Autodesk Inventor part; units mm, degrees
ref_plane "YZ Plane" through (0, 0, 0) normal (1, 0, 0) x (0, 1, 0)
ref_plane "XZ Plane" through (0, 0, 0) normal (0, 1, 0) x (-1, 0, 0)
ref_plane "XY Plane" through (0, 0, 0) normal (0, 0, 1) x (1, 0, 0)
sketch "Sketch1" plane through (0, 0, 0) normal (0, 0, 1) x (1, 0, 0)
  line L0 (21.5871, 13.6345) -> (17.0871, 18.1345)
  line L1 (17.0871, 18.1345) -> (-16.7129, 18.1345)
  line L2 (-16.7129, 18.1345) -> (-21.2129, 13.6345)
  line L3 (-21.0966, 13.6345) -> (-21.0966, -20.1655)
  line L4 (21.4709, -20.1655) -> (21.4709, 13.6345)
  line L5 (21.4709, -20.1655) -> (17.0871, -24.4078)
  line L6 (-16.7129, -24.4078) -> (17.0871, -24.4078)
  line L7 (-16.7129, -24.4078) -> (-21.0966, -20.1655)
  line L8 (-24.7129, -28.1655) -> (-24.7129, 13.6345) construction
  line L9 (25.0871, -28.1655) -> (-24.7129, -28.1655) construction
  line L10 (25.0871, -28.1655) -> (25.0871, 13.6345) construction
  line L11 (17.0871, 21.6345) -> (-16.7129, 21.6345) construction
  line L12 (-21.0552, -20.0655) -> (-16.6129, -24.5078)
  line L13 (-16.6129, -24.5078) -> (-16.6129, -28.1655)
  line L14 (-16.6129, -28.1655) -> (17.0871, -28.1655)
  line L15 (25.0871, -20.0655) -> (21.4295, -20.0655)
  line L16 (25.0871, 13.5345) -> (25.0871, -20.0655)
  line L17 (21.4295, 13.5345) -> (25.0871, 13.5345)
  line L18 (21.4295, 13.5345) -> (16.9871, 17.9768)
  line L19 (16.9871, 17.9768) -> (16.9871, 21.6345)
  line L20 (16.9871, 21.6345) -> (-16.6129, 21.6345)
  line L21 (-16.6129, 21.6345) -> (-16.6129, 17.9768)
  line L22 (-16.6129, 17.9768) -> (-21.0552, 13.5345)
  line L23 (-24.7129, 13.5345) -> (-21.0552, 13.5345)
  line L24 (-24.7129, -20.0655) -> (-24.7129, 13.5345)
  line L25 (-21.0552, -20.0655) -> (-24.7129, -20.0655)
  line L26 (-12.3129, -23.2655) -> (12.6871, -23.2655)
  line L27 (12.6871, -23.2655) -> (12.6871, 16.7345)
  line L28 (-12.3129, 16.7345) -> (12.6871, 16.7345)
  line L29 (-12.3129, -23.2655) -> (-12.3129, 16.7345)
  line L30 (14.6871, -25.2655) -> (-14.3129, -25.2655) construction
  line L31 (-14.3129, -25.2655) -> (-14.3129, 18.7345) construction
  line L32 (-14.3129, 18.7345) -> (14.6871, 18.7345) construction
  line L33 (14.6871, 18.7345) -> (14.6871, -25.2655) construction
  line L34 (-17.3129, 21.7345) -> (17.6871, 21.7345) construction
  line L35 (17.6871, 21.7345) -> (17.6871, -28.2655) construction
  line L36 (17.6871, -28.2655) -> (-17.3129, -28.2655) construction
  line L37 (-17.3129, -28.2655) -> (-17.3129, 21.7345) construction
  line L38 (-14.3129, -23.2655) -> (-14.3129, -25.2655)
  line L39 (-14.3129, -25.2655) -> (14.6871, -25.2655)
  line L40 (14.6871, -25.2655) -> (14.6871, -20.0655)
  line L41 (14.6871, -20.0655) -> (17.6871, -20.0655)
  line L42 (17.6871, -20.0655) -> (17.6871, 13.5345)
  line L43 (17.6871, 13.5345) -> (14.6871, 13.5345)
  line L44 (14.6871, 13.5345) -> (14.6871, 18.7345)
  line L45 (14.6871, 18.7345) -> (-14.3129, 18.7345)
  line L46 (-14.3129, 18.7345) -> (-14.3129, 13.5345)
  line L47 (-14.3129, 13.5345) -> (-17.3129, 13.5345)
  line L48 (-17.3129, 13.5345) -> (-17.3129, -20.0655)
  line L49 (-17.3129, -20.0655) -> (-14.3129, -20.0655)
  line L50 (-14.3129, -20.0655) -> (-14.3129, -23.2655)
  line L51 (-16.6129, -28.1655) -> (17.0871, -28.1655)
  line L52 (16.9871, -28.1655) -> (16.9871, -24.3509)
  line L53 (16.9871, -24.3509) -> (21.2726, -20.0655)
  line L54 (21.2726, -20.0655) -> (21.4295, -20.0655)
  point P0 (14.2, -44.8454)
  point P1 (16.9871, 19.8057)
  dimension "d74" = 2
  dimension "d75" = 5
  dimension "d76" = 135
extrude "Extrusion1" add sketch "Sketch1" along normal blind 8 contours L19 L18 L17 L4 L15 L54 L53 L52 L6 L40 L41 L42 L43 L44 L1 | L1 L44 L45 L46 L21 L20 L19 | L44 L43 L42 L41 L40 L6 L38 L50 L49 L48 L47 L46 L1 | L1 L46 L45 L44 | L46 L47 L48 L49 L50 L38 L6 L12 L25 L3 L23 L22 L21 L1 | L17 L16 L15 L4 | L3 L25 L24 L23 | L40 L39 L38 L6 | L6 L52 L14 L13 L12 L38 L39 L40 | L29 L28 L27 L26
sketch "Skizze7" plane through (0, 0, 8) normal (0, 0, 1) x (1, 0, 0)
  line L0 (-21.0552, -20.0655) -> (-16.6129, -24.5078)
  line L1 (-16.6129, -24.5078) -> (-16.6129, -28.1655)
  line L2 (-16.6129, -28.1655) -> (16.9871, -28.1655) construction
  line L3 (16.9871, -28.1655) -> (16.9871, -24.3509)
  line L4 (16.9871, -24.3509) -> (21.2726, -20.0655)
  line L5 (21.2726, -20.0655) -> (25.0871, -20.0655)
  line L6 (25.0871, -20.0655) -> (25.0871, 13.5345) construction
  line L7 (25.0871, 13.5345) -> (21.4295, 13.5345)
  line L8 (21.4295, 13.5345) -> (16.9871, 17.9768)
  line L9 (16.9871, 17.9768) -> (16.9871, 21.6345)
  line L10 (16.9871, 21.6345) -> (-16.6129, 21.6345) construction
  line L11 (-16.6129, 21.6345) -> (-16.6129, 17.9768)
  line L12 (-16.6129, 17.9768) -> (-21.0552, 13.5345)
  line L13 (-21.0552, 13.5345) -> (-24.7129, 13.5345)
  line L14 (-24.7129, 13.5345) -> (-24.7129, -20.0655) construction
  line L15 (-24.7129, -20.0655) -> (-21.0552, -20.0655)
  line L16 (-16.8129, 21.8345) -> (17.1871, 21.8345) construction
  line L17 (17.1871, 21.8345) -> (17.1871, 18.0597)
  line L18 (17.1871, 18.0597) -> (21.5123, 13.7345)
  line L19 (21.5123, 13.7345) -> (25.2871, 13.7345)
  line L20 (25.2871, 13.7345) -> (25.2871, -20.2655) construction
  line L21 (25.2871, -20.2655) -> (21.3554, -20.2655)
  line L22 (21.3554, -20.2655) -> (17.1871, -24.4338)
  line L23 (17.1871, -24.4338) -> (17.1871, -28.3655)
  line L24 (17.1871, -28.3655) -> (-16.8129, -28.3655) construction
  line L25 (-16.8129, -28.3655) -> (-16.8129, -24.5907)
  line L26 (-16.8129, -24.5907) -> (-21.1381, -20.2655)
  line L27 (-21.1381, -20.2655) -> (-24.9129, -20.2655)
  line L28 (-24.9129, -20.2655) -> (-24.9129, 13.7345) construction
  line L29 (-24.9129, 13.7345) -> (-21.1381, 13.7345)
  line L30 (-21.1381, 13.7345) -> (-16.8129, 18.0597)
  line L31 (-16.8129, 18.0597) -> (-16.8129, 21.8345)
  line L32 (-21.0552, 13.5345) -> (-24.7129, 13.5345)
  line L33 (-24.7129, 13.5345) -> (-24.7129, 13.7345)
  line L34 (-16.6129, 21.6345) -> (-16.6129, 17.9768)
  line L35 (-16.6129, 21.6345) -> (-16.8129, 21.6345)
  line L36 (25.0871, -20.0655) -> (25.0871, 13.5345)
  line L37 (25.0871, 13.5345) -> (25.0871, 13.7345)
  line L38 (16.9871, 21.6345) -> (17.1871, 21.6345)
  line L39 (16.9871, -28.1655) -> (17.1871, -28.1655)
  line L40 (25.0871, -20.0655) -> (25.0871, -20.2655)
  line L41 (-16.6129, -28.1655) -> (-16.8129, -28.1655)
  line L42 (-24.7129, -20.0655) -> (-24.7129, -20.2655)
  dimension "d94" = 0.2
extrude "IM_offset" add sketch "Skizze7" against normal up to surface (8 mm away)
sketch "Sketch8" plane through (-1.6003, 36.8471, 0) normal (0.7071, 0.7071, 0) x (0.7071, -0.7071, 0)
  arc A0 (21.9778, -0.9777) -> (37.2778, -0.9777) centre (29.6278, -0.9777) ccw
  line L0 (21.9778, -0.9777) -> (37.2778, -0.9777) construction
  line L1 (21.9778, -0.9777) -> (37.2778, -0.9777) construction
  line L2 (21.9778, -0.9777) -> (37.2778, -0.9777)
  point P0 (27.1864, 0)
  point P1 (29.6278, -1.0154)
  dimension "d98" = 15.3
  dimension "d99" = 0
  dimension "d100" = 7.65
extrude "Extrusion7" cut sketch "Sketch8" against normal blind 45 and the other way blind 22.5
sketch "Sketch9" plane through (0, 0, 8) normal (0, 0, 1) x (1, 0, 0)
  line L0 (17.1871, 21.6345) -> (-16.8129, 21.6345)
  line L1 (-24.7129, 13.7345) -> (-24.7129, -20.2655)
  line L2 (17.1871, -28.1655) -> (-16.8129, -28.1655)
  line L3 (25.0871, -20.0655) -> (25.0871, 13.7345)
  circle A0 centre (0.1871, -3.187) radius 27.0445
  circle A1 centre (0.1871, -3.187) radius 15
  line L4 (-16.8129, 21.6345) -> (-16.8129, 18.0597)
  line L5 (-16.8129, 18.0597) -> (-21.1381, 13.7345)
  line L6 (-21.1381, 13.7345) -> (-24.7129, 13.7345)
  line L7 (17.1871, -28.1655) -> (17.1871, -24.4338)
  line L8 (17.1871, -24.4338) -> (21.3554, -20.2655)
  line L9 (21.3554, -20.2655) -> (25.0871, -20.2655)
  line L10 (25.0871, -20.2655) -> (25.0871, -20.0655)
  line L11 (25.0871, 13.7345) -> (21.5123, 13.7345)
  line L12 (21.5123, 13.7345) -> (21.4956, 13.7512)
  line L13 (17.1871, 18.0597) -> (17.1871, 21.6345)
  line L14 (-21.1381, -20.2655) -> (-24.7129, -20.2655)
  line L15 (-16.8129, -24.5907) -> (-21.1381, -20.2655)
  line L16 (-16.8129, -28.1655) -> (-16.8129, -24.5907)
  line L17 (21.4956, 13.7512) -> (-10.3242, -18.0686)
  line L18 (-10.3242, -18.0686) -> (-14.6159, -13.7769)
  line L19 (-14.6159, -13.7769) -> (17.2039, 18.043)
  line L20 (17.2039, 18.043) -> (17.1871, 18.0597)
  point P0 (0, 0)
  dimension "d91" = 30
extrude "Extrusion8" cut sketch "Sketch9" against normal through all contours L19 A1 | A1 L17 L19 | A1 L17
sketch "Sketch10" plane through (21.5123, 13.7345, 1.6478) normal (0.7071, 0.7071, 0) x (0, 0, -1)
  line L0 (-6.3522, 0.0237) -> (-6.3522, 6.0931)
  arc A0 (-6.3522, 0.0237) -> (0.6701, -4.5916) centre (0.6701, 3.0584) ccw
  line L1 (0.6701, 10.7084) -> (0.6701, -4.5916)
  arc A1 (0.6701, 10.7084) -> (-6.3522, 6.0931) centre (0.6701, 3.0584) ccw
  point P0 (1.6478, 5.4998)
properties part number "20_Cube_Insert_Lens_Cylindrical_v3"
Geometry: final body of the model. Coordinates: model frame, mm. A direction names the side the tool comes from. Round coordinates to 2 decimals unless told otherwise and drop trailing zeros. Write each loop counter-clockwise with the first axis right and the second up, starting at its lowest first coordinate (ties: lowest second). Pieces come first, ordered by that corner, then holes.
Item 1: Set-up query: faces 1 (the face through (23, -20.266, 4)), 2 (the face through (24.1, 13.734, 7.5)), 3 (the face through (-6.551, -18.996, 5.231)). Return all of +Z, -Z, +X, -X, +Y, -Y with unobstructed straight access to the full face (end or side cutting, diameter ignored); none if empty.
Item 2: Section query A-A (y = -1.5). Return loops of the section in (x, z), plus the area to 3 significant figures.
Item 3: Section query D-D (z = 2). Return loops of the section in (x, y), plus the area to 3 significant figures.
Item 4: Section query C-C (z = 5.5). Return loops of the section in (x, y), plus the area to 3 significant figures.
Item 5: Material intervals for L1, parallel to Z at x = 20.5, y = 7.5; L2, parallel to Y at x = 12.5, z = 3.25; L3, parallel to Y at x = 5.5, z = 6, sorted ascending.
Item 6: Pin query (flat end, axial travel): P1, Ø0.8, axis at x = 24, z = 0.5, coming from the +Y side; P2, Ø1.8, axis at x = -23, z = 2, coming from the -Y side; P3, Ø0.8, axis at y = 19, z = 0.5, coming from the +X side; P4, Ø24, axis at x = 0.19, y = -3.19, coming from the +Z side. Return the tip coordinate at first contact, or that it passes through.
Item 7: Mould query, pull axis X, two halves, no side actions, for faces 4 (the face through (-15.61, -9.974, 5.127)), 5 (the face through (-16.813, 20, 4)), 6 (the face through (0, -28.166, 4)). Classes: +X half, -X half, draft (parallel to the pull), parting line (faces both ways), or undercut.
Item 8: Section query B-B (x = 2.5). Return loops of the section in (y, z), plus the area to 3 significant figures.
Completed:
1. face 1: +Z, -Z, +X, -Y
1. face 2: +Z, -Z, +X, +Y
1. face 3: none
2. outline: (-24.71, 0) - (-14.72, 0) - (-14.72, 8) - (-24.71, 8) - close; (15.09, 0) - (25.09, 0) - (25.09, 8) - (15.09, 8) - close
2. area: 160 mm2
3. outline: (-24.71, -20.27) - (-21.14, -20.27) - (-16.81, -24.59) - (-16.81, -28.17) - (17.19, -28.17) - (17.19, -24.43) - (21.36, -20.27) - (25.09, -20.27) - (25.09, 10.91) - (14.72, 0.54) arc R15 cw to (-3.54, -17.72) - (-7.11, -21.28) - (-17.83, -10.56) - (-14.31, -7.04) arc R15 cw to (4.04, 11.31) - (14.37, 21.63) - (-16.81, 21.63) - (-16.81, 18.06) - (-21.14, 13.73) - (-24.71, 13.73) - close
3. area: 1,300 mm2
4. outline: (-24.71, -20.27) - (-21.14, -20.27) - (-16.81, -24.59) - (-16.81, -28.17) - (17.19, -28.17) - (17.19, -24.43) - (21.36, -20.27) - (25.09, -20.27) - (25.09, 12.91) - (14.24, 2.06) arc R15 cw to (-5.06, -17.24) - (-8.11, -20.29) - (-16.83, -11.56) - (-13.82, -8.55) arc R15 cw to (5.55, 10.82) - (16.36, 21.63) - (-16.81, 21.63) - (-16.81, 18.06) - (-21.14, 13.73) - (-24.71, 13.73) - close
4. area: 1,360 mm2
5. L1: z = 0 to 0.98, 4.58 to 8
5. L2: y = -28.17 to -11.75, 19.38 to 21.63
5. L3: y = -28.17 to -17.21, 10.84 to 21.63
6. P1: stops at y = 13.73
6. P2: stops at y = -20.27
6. P3: stops at x = 17.19
6. P4: passes through
7. face 4: undercut
7. face 5: -X half
7. face 6: draft
8. outline: (-28.17, 0) - (-18.01, 0) - (-18.01, 8) - (-28.17, 8) - close; (11.63, 0) - (21.63, 0) - (21.63, 8) - (11.63, 8) - close
8. area: 161 mm2
